Geometry check sheet. Reference: the model listing, model coordinates, mm. Face numbers are marked on the shaded views. A direction names the side the tool comes from. Round coordinates to 2 decimals unless told otherwise and drop trailing zeros. Order: outer loops, then holes, each group sorted by start corner. A loop starts at its lowest first (then second) coordinate and runs counter-clockwise, first axis right, second up. Notation, with made-up numbers: M 76.5,54.5 L 127.5,54.5 A28 ccw 127.5,88.5 Z; hole C -29.75,25.25 d7. An arc over 180 degrees is marked long. Answer as a JSON object with one key per item and string values. Group by question number.
```python
from build123d import *

# Parameters (mm, degrees)
SKETCH1_R      = 4
EXTRUDE1_DEPTH = 13
FILLET5_R      = 5
FILLET6_R      = 5
SKETCH8_R      = 4
EXTRUDE7_DEPTH = 30


with BuildPart() as part:
    # Sketch1 → Extrude1 (new body)
    with BuildSketch(Plane(origin=(0, 0, 0), x_dir=(1, 0, 0), z_dir=(0, 1, 0))):
        Polygon((0, -15), (-15, 0), (-22, 0), (-22, 30), (-2.573593129, 30), (30, -2.573593129), (30, -42), (0, -42), align=None)
        with Locations((-8.786796564, 15)):
            Circle(SKETCH1_R, mode=Mode.SUBTRACT)
        with Locations((15, -8.786796564)):
            Circle(SKETCH1_R, mode=Mode.SUBTRACT)
    extrude(amount=EXTRUDE1_DEPTH)

    # Fillet5
    fillet5_edges = [part.edges().sort_by_distance(p)[0] for p in [
        (-2.573593129, 6.5, -30),
        (30, 6.5, 2.573593129),
        (30, 6.5, 42),
        (0, 6.5, 42),
        (0, 6.5, 15),
        (-15, 6.5, 0),
    ]]
    fillet(fillet5_edges, radius=FILLET5_R)

    # Fillet6
    fillet6_edges = [part.edges().sort_by_distance(p)[0] for p in [
        (-22, 6.5, 0),
        (-22, 6.5, -30),
    ]]
    fillet(fillet6_edges, radius=FILLET6_R)

    # Sketch8 → Extrude7 (cut)
    with BuildSketch(Plane.ZY):
        with Locations((28, 6.5)):
            Circle(SKETCH8_R)
    extrude(amount=-EXTRUDE7_DEPTH, mode=Mode.SUBTRACT)


solid = part.part
```
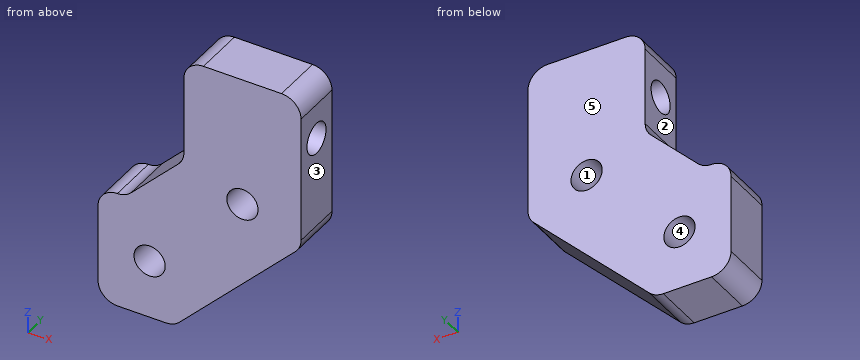
1) Sectioned sample at B-B (z = 28). Record the boundary of the cut face in (x, y), then the cut area to 3 significant figures.
2) Thickness scan on line 1 along Z through (x, y) = (16.5, 3.75); line 2 along Y through (x, z) = (11, 28); line 3 along Z through (x, y) = (15, 7.25). Record the ranges inside material, lowest first. Write a range as [from, to].
3) Release check for a two-part mould opening along X. For the marked faces 3, 4 and 5 record: +X half, -X half, draft (parallel to the pull), parting line (faces both ways), or undercut.
4) Set-up check for the marked faces 1 and 2: record each of +Z, -Z, +X, -X, +Y, -Y from which the full face is reachable in a straight line by a thin tool's end or side.
5) Go/stop test with flat-tipped pins: P1, Ø2, axis at x = -12.5, y = 2, coming from the +Z side; P2, Ø6.5, axis at x = 15, z = 8.79, coming from the +Y side; P3, Ø6.5, axis at y = 5.5, z = 24, coming from the -X side; P4, Ø6, axis at y = 8.5, z = 16, coming from the -X side. Record where each tip stops, or that it passes through.
6) Sectioned sample at A-A (x = 15). Record the boundary of the cut face in (y, z), then the cut area to 3 significant figures.
7) Sectioned sample at C-C (y = 6.5). Count the separate pieces of the cut face and the enclosed holes in it, then the cut area to 3 significant figures.
8) Sectioned sample at D-D (x = -6). Record the boundary of the cut face in (y, z).
Final values:
{
 "1": {"outline": "M 0,0 L 30,0 L 30,2.5 L 0,2.5 Z; M 0,10.5 L 30,10.5 L 30,13 L 0,13 Z", "area": "150 mm^2"},
 "2": {"line 1": "z = [-10.93, 5.08], [12.49, 25.1], [30.9, 42]", "line 2": "y = [0, 2.5], [10.5, 13]", "line 3": "z = [-12.43, 4.79], [12.79, 24.07], [31.93, 42]"},
 "3": {"face 3": "+X half", "face 4": "undercut", "face 5": "draft"},
 "4": {"face 1": "+Y, -Y", "face 2": "+Z, -X, +Y, -Y"},
 "5": {"P1": "stops at z = 3.5", "P2": "passes through", "P3": "stops at x = 0", "P4": "stops at x = -2"},
 "6": {"outline": "M 0,-12.43 L 13,-12.43 L 13,4.79 L 0,4.79 Z; M 0,12.79 L 13,12.79 L 13,42 L 0,42 Z; hole C 6.5,28 d8", "area": "553 mm^2"},
 "7": {"separate pieces": "2", "enclosed holes": "2", "area": "2,040 mm^2"},
 "8": {"outline": "M 0,-30 L 13,-30 L 13,-17.87 L 0,-17.87 Z; M 0,-12.13 L 13,-12.13 L 13,9 L 0,9 Z"}
}
